Verification items for the finished model (mm, model axes). A direction names the side the tool comes from. Round coordinates to 2 decimals unless told otherwise and drop trailing zeros. Write each loop counter-clockwise with the first axis right and the second up, starting at its lowest first coordinate (ties: lowest second). Pieces come first, ordered by that corner, then holes. Notation, with made-up numbers: (12.5, 69.25) -> (41.5, 69.25) arc R29 ccw to (41.5, 107.25) -> close; hole circle Ø4 at (26, 46.25). An arc over 180 degrees is marked (long way). Answer as a JSON object with one key per item and string values. Group by question number.
(1) Scan lines: L1, parallel to Y at x = -18.5, z = -10.5; L2, parallel to Z at x = -16, y = 44; L3, parallel to Y at x = -6, z = -43.5. Record each from-to range of solid material in increasing order. Write a range as from..to.
(2) Gauge pin test, flat ends, axial feed: pin 1 Ø1.6 at (x, z) = (-0.5, 43.5) entering from +Y; pin 2 Ø12 at (x, z) = (-24.5, 11) entering from +Y; pin 3 Ø4 at (y, z) = (-35, 0.5) entering from -X; pin 4 Ø3 at (x, z) = (-8, -44) entering from -Y. Record the tip position at first contact, or that the pin passes through.
(3) Set-up check for faces 5 (the face through (-60, 0, 18)), 6 (the face through (-6.383, -60.208, -44.67)), 7 (the face through (-59.486, 1.308, -24.65)): record each of +Z, -Z, +X, -X, +Y, -Y from which the full face is reachable in a straight line by a thin tool's end or side.
(4) Draft check along Y on faces 1 (the face through (-1.999, -44, 46)), 2 (the face through (-60, -5, 8)), 3 (the face through (-39, -3, 50)), 4 (the face through (-61.985, 1.363, -25.35)). Enter one of: released by +Y, released by -Y, zero draft, split by the parting line, or undercut.
(5) Sectioned sample at A-A on z = -44. Record the cut outline in (x, y).
(6) Sectioned sample at C-C on z = -32. Record the cut outline in (x, y).
(7) Sectioned sample at B-B on x = -8. Count the separate pieces of the cut face and the enclosed holes in it, and give its area (3 significant figures).
```python
from build123d import *

# Parameters (mm, degrees)
F1_ANGLE_BACK = 90
F1_ANGLE      = 180
F3_DEPTH      = 49
F4_DEPTH      = 42
F5_DEPTH      = 53
F6_R          = 1.75
F7_DEPTH      = 62.5
F8_W          = 10
F8_H          = 20
F8_R          = 1.5
F9_DEPTH      = 62.0010001


with BuildPart() as f1:
    # F0 (on Front) → F1 (revolve)
    with BuildSketch(Plane.XZ, mode=Mode.PRIVATE) as f1_sk:
        with BuildLine():
            ThreePointArc((-35.5, 47), (-36.3786796564, 49.1213203436), (-38.5, 50))
            Line((-38.5, 50), (-49, 50))
            add(Edge.make_bspline(
                [(-49, 50), (-50.0905438599, 49.4592544488), (-53.0493875637, 47.4989733534), (-57.4486951492, 41.931344871), (-61.5763053799, 28.0443008729), (-61.4881986154, 14.5014666819), (-62, 0)],
                knots=[0, 0, 0, 0, 0.1531073754, 0.3436852098, 0.6019385566, 1, 1, 1, 1], degree=3))
            Line((-62, 0), (-62, -50))
            Line((-62, -50), (-59.5, -50))
            Line((-59.5, -50), (-59.5, 0))
            add(Edge.make_bspline(
                [(-51.1955396277, 43), (-59.7999691963, 32.3488041759), (-58.4857873619, 15.5563373119), (-59.5, 0)],
                knots=[0, 0, 0, 0, 43.7945665817, 43.7945665817, 43.7945665817, 43.7945665817], degree=3))
            Line((-51.1955396277, 43), (-38.5, 43))
            ThreePointArc((-38.5, 43), (-36.3786796564, 43.8786796564), (-35.5, 46))
            Line((-35.5, 46), (-35.5, 47))
        make_face()
    revolve(f1_sk.sketch.rotate(Axis((0, 0, -47.5967168808), (0, 0, 1)), -F1_ANGLE_BACK), axis=Axis((0, 0, -47.5967168808), (0, 0, 1)), revolution_arc=F1_ANGLE)

    # F2 (on Front) → F3 (cut)
    with BuildSketch(Plane.XZ):
        with BuildLine():
            ThreePointArc((0, 45), (1.4142135624, 45.5857864376), (2, 47))
            ThreePointArc((2, 47), (1.4142135624, 48.4142135624), (0, 49))
            ThreePointArc((0, 49), (-1.3909130574, 48.4371363424), (-1.998931704, 47.0653608667))
            Line((-1.998931704, 47.0653608667), (-1.998931704, 46.9346391333))
            ThreePointArc((-1.998931704, 46.9346391333), (-1.3909130574, 45.5628636576), (0, 45))
        make_face()
    extrude(amount=F3_DEPTH, mode=Mode.SUBTRACT)

    # F2 (on Front) → F4 (cut)
    with BuildSketch(Plane.XZ):
        with BuildLine():
            ThreePointArc((-1.998931704, 47.0653608667), (-1.3909130574, 48.4371363424), (0, 49))
            Line((0, 49), (0, 50.3604523001))
            Line((0, 50.3604523001), (-1.998931704, 50.3604523001))
            Line((-1.998931704, 50.3604523001), (-1.998931704, 47.0653608667))
        make_face()
    extrude(amount=F4_DEPTH, mode=Mode.SUBTRACT)

    # F2 (on Front) → F5 (cut)
    with BuildSketch(Plane.XZ):
        with BuildLine():
            Line((0, 41.0653608667), (0, 45))
            ThreePointArc((0, 45), (-1.3909130574, 45.5628636576), (-1.998931704, 46.9346391333))
            Line((-1.998931704, 46.9346391333), (-1.998931704, 41.0653608667))
            Line((-1.998931704, 41.0653608667), (0, 41.0653608667))
        make_face()
    extrude(amount=F5_DEPTH, mode=Mode.SUBTRACT)

    # F6 (on Front) → F7 (cut, symmetric)
    with BuildSketch(Plane.XZ):
        with Locations((-8, -44)):
            Circle(F6_R)
    extrude(amount=F7_DEPTH, both=True, mode=Mode.SUBTRACT)

    # F8 (on Right) → F9 (cut, through all)
    with BuildSketch(Plane.YZ):
        with Locations((0, 8)):
            Rectangle(F8_W, F8_H)
        with Locations((-12.5, 19)):
            Circle(F8_R)
        with Locations((12.5, 19)):
            Circle(F8_R)
        with Locations((12.5, -1)):
            Circle(F8_R)
        with Locations((-12.5, -1)):
            Circle(F8_R)
    extrude(amount=-F9_DEPTH, mode=Mode.SUBTRACT)


solid = f1.part
```
Computed values:
{
 "1": {"L1": "-59.18..-56.55, 56.55..59.18", "L2": "43..50", "L3": "-61.71..-59.2, 59.2..61.71"},
 "2": {"pin 1": "y = 56.37", "pin 2": "y = 58.83", "pin 3": "x = -52.47", "pin 4": "through"},
 "3": {"face 5": "+X, -X", "face 6": "+Y, -Y", "face 7": "-Z, +X"},
 "4": {"face 1": "undercut", "face 2": "undercut", "face 3": "zero draft", "face 4": "split by the parting line"},
 "5": {"outline": "(-9.75, -61.23) -> (-9.75, -58.7) arc R59.5 cw to (-9.75, 58.7) -> (-9.75, 61.23) arc R62 ccw to start; (-6.25, -61.68) arc R62 ccw to (0, -62) -> (0, -59.5) arc R59.5 cw to (-6.25, -59.17) -> close; (-6.25, 59.17) arc R59.5 cw to (0, 59.5) -> (0, 62) arc R62 ccw to (-6.25, 61.68) -> close"},
 "6": {"outline": "(0, -62) -> (0, -59.5) arc R59.5 cw to (0, 59.5) -> (0, 62) arc R62 ccw to start"},
 "7": {"separate pieces": "4", "enclosed holes": "0", "area": "752 mm2"}
}
